from build123d import *

# Parameters (mm, degrees)
SKETCH1_R           = 1.25
SKETCH1_W           = 1
SKETCH1_H           = 4
BOSS_EXTRUDE1_DEPTH = 5
SKETCH3_R           = 1.5
CUT_EXTRUDE1_DEPTH  = 4


with BuildPart() as part:
    # Sketch1 → Boss-Extrude1 (new body)
    with BuildSketch(Plane(origin=(0, 0, 0), x_dir=(1, 0, 0), z_dir=(0, 1, 0))):
        with BuildLine():
            Line((-13, -3), (-13, -12))
            Line((-13, -12), (-9, -12))
            Line((-9, -12), (-9, -5))
            ThreePointArc((-9, -5), (-8.707106781, -4.292893219), (-8, -4))
            Line((-8, -4), (12, -4))
            ThreePointArc((12, -4), (12.707106781, -3.707106781), (13, -3))
            Line((13, -3), (13, 3))
            ThreePointArc((13, 3), (12.707106781, 3.707106781), (12, 4))
            Line((12, 4), (-8, 4))
            ThreePointArc((-8, 4), (-8.707106781, 4.292893219), (-9, 5))
            Line((-9, 5), (-9, 12))
            Line((-9, 12), (-13, 12))
            Line((-13, 12), (-13, 4))
            Line((-13, 4), (-13, -3))
        make_face()
        with Locations(Location((10, 0, 0), (0, 0, 270))):
            Circle(SKETCH1_R, mode=Mode.SUBTRACT)
        with Locations(Location((-9, 0, 0), (0, 0, 270))):
            Circle(SKETCH1_R, mode=Mode.SUBTRACT)
        with Locations((4.3, 0)):
            Rectangle(SKETCH1_W, SKETCH1_H, mode=Mode.SUBTRACT)
        with Locations((-3.3, 0)):
            Rectangle(SKETCH1_W, SKETCH1_H, mode=Mode.SUBTRACT)
    extrude(amount=BOSS_EXTRUDE1_DEPTH)

    # Sketch3 → Cut-Extrude1 (cut)
    with BuildSketch(Plane.ZY.offset(13)):
        with Locations((9, 2.5)):
            Circle(SKETCH3_R)
        with Locations((-9, 2.5)):
            Circle(SKETCH3_R)
    extrude(amount=-CUT_EXTRUDE1_DEPTH, mode=Mode.SUBTRACT)


solid = part.part
Model file for the job. Use its own axes, mm. A direction names the side the tool comes from. Coordinates: 2 decimals unless noted, no trailing zeros. Order: outer loops, then holes, each group sorted by start corner. A loop starts at its lowest first (then second) coordinate and runs counter-clockwise, first axis right, second up. Notation, with made-up numbers: (-9.75, -10) -> (19.25, -10) arc R32 ccw to (19.25, 18) -> close; hole circle Ø1 at (78, 39.25). An arc over 180 degrees is marked (long way). Return JSON: item names as keys, results as strings. Group by question number.
Item 1: Saw through at C-C on x = 10. Write the cut outline in (y, z), then the cut area to 3 significant figures.
Item 2: Wall check: line 1 along X through (y, z) = (3.9, 0); line 2 along X through (y, z) = (2, 1.5); line 3 along Z through (x, y) = (-3.75, 3.7). Give the ranges that are in metal, low to high. Write a range as [from, to].
Item 3: Pull direction X, two halves, no side cores. Call faces 4 (the flat face through (3.8, 2, 0)), 5 (the flat face through (-9, 1, 8)), 6 (the flat face through (2, 2, 4)): pulls with the +X half, pulls with the -X half, needs draft (parallel to the pull), parting line crosses it, or undercut.
Item 4: Tool access for faces 1 (the flat face through (-3, 2, -2)), 2 (the flat face through (2, 2, -4)), 3 (the flat face through (-11, 2, -12)): list every direction of +Z, -Z, +X, -X, +Y, -Y with a clear straight run to the whole face (end or side of a thin tool).
Item 5: Saw through at D-D on z = 0. Write the cut outline in (x, y), then the cut area to 3 significant figures.
Item 6: Flat gauge pins, fed straight in: P1, Ø1.1, axis at x = 4, y = 3, coming from the -Z side; P2, Ø1.1, axis at x = 4.5, y = 1.5, coming from the +Z side; P3, Ø1.5, axis at y = 2, z = 7.5, coming from the +X side. Where does each tip first touch, or does it go through?
Item 7: Saw through at A-A on y = 3.4. State how many separate pieces and enclosed holes the cut face has, then the cut area to 3 significant figures.
Item 8: Saw through at B-B on z = -9. Write the cut outline in (x, y), then the cut area to 3 significant figures.
Values found:
{
 "1": {"outline": "(0, -4) -> (5, -4) -> (5, -1.25) -> (0, -1.25) -> close; (0, 1.25) -> (5, 1.25) -> (5, 4) -> (0, 4) -> close", "area": "27.5 mm2"},
 "2": {"line 1": "x = [-13, -10.25], [-7.75, -3.8], [-2.8, 3.8], [4.8, 8.75], [11.25, 13]", "line 2": "x = [-13, -3.8], [-2.8, 3.8], [4.8, 13]", "line 3": "z = [-4, -2], [2, 4]"},
 "3": {"face 4": "undercut", "face 5": "pulls with the +X half", "face 6": "needs draft"},
 "4": {"face 1": "+Y, -Y", "face 2": "-Z, +X, +Y, -Y", "face 3": "-Z, +X, -X, +Y, -Y"},
 "5": {"outline": "(-13, 0) -> (-10.25, 0) -> (-10.25, 5) -> (-13, 5) -> close; (-7.75, 0) -> (-3.8, 0) -> (-3.8, 5) -> (-7.75, 5) -> close; (-2.8, 0) -> (3.8, 0) -> (3.8, 5) -> (-2.8, 5) -> close; (4.8, 0) -> (8.75, 0) -> (8.75, 5) -> (4.8, 5) -> close; (11.25, 0) -> (13, 0) -> (13, 5) -> (11.25, 5) -> close", "area": "95.0 mm2"},
 "6": {"P1": "stops at z = -4", "P2": "stops at z = 4", "P3": "stops at x = -9"},
 "7": {"separate pieces": "3", "enclosed holes": "4", "area": "235 mm2"},
 "8": {"outline": "(-13, 0) -> (-9, 0) -> (-9, 1) -> (-13, 1) -> close; (-13, 4) -> (-9, 4) -> (-9, 5) -> (-13, 5) -> close", "area": "8.00 mm2"}
}
